Autodesk Inventor part; units mm, degrees
ref_plane "YZ Plane" through (0, 0, 0) normal (1, 0, 0) x (0, 1, 0)
ref_plane "XZ Plane" through (0, 0, 0) normal (0, 1, 0) x (-1, 0, 0)
ref_plane "XY Plane" through (0, 0, 0) normal (0, 0, 1) x (1, 0, 0)
sketch "Sketch1" plane through (0, 0, 0) normal (0, 1, 0) x (-1, 0, 0)
  line L0 (9.1683, 14.0813) -> (-48.6317, 14.0813)
  line L1 (-48.6317, 14.0813) -> (-48.6317, -63.9187)
  line L2 (-48.6317, -63.9187) -> (9.1683, -63.9187)
  line L3 (9.1683, -63.9187) -> (9.1683, 14.0813)
  point P0 (0, 0)
  dimension "d0" = 57.8
  dimension "d1" = 78
extrude "Extrusion1" add sketch "Sketch1" along normal blind 2
sketch "Sketch2" plane through (0, 2, 0) normal (0, 1, 0) x (1, 0, 0)
  line L0 (-9.1683, 63.9187) -> (-9.1683, -14.0813)
  line L1 (48.6317, 63.9187) -> (-9.1683, 63.9187)
  line L2 (-9.1683, -14.0813) -> (-1.1683, -14.0813)
  line L3 (-1.1683, -14.0813) -> (-1.1683, 63.9187)
  line L4 (-1.1683, 63.9187) -> (-9.1683, 63.9187)
  line L5 (-9.1683, 63.9187) -> (-9.1683, -14.0813)
  line L6 (48.6317, -14.0813) -> (48.6317, 63.9187)
  line L7 (48.6317, -14.0813) -> (40.6317, -14.0813)
  line L8 (40.6317, -14.0813) -> (40.6317, 63.9187)
  line L9 (40.6317, 63.9187) -> (48.6317, 63.9187)
  line L10 (48.6317, 63.9187) -> (48.6317, -14.0813)
  line L11 (1.2317, -14.0813) -> (1.2317, 63.9187)
  line L12 (-9.1683, -14.0813) -> (48.6317, -14.0813)
  line L13 (38.2317, -14.0813) -> (38.2317, 63.9187)
  line L14 (1.2317, -14.0813) -> (38.2317, -14.0813)
  line L15 (1.2317, 63.9187) -> (38.2317, 63.9187)
  point P0 (0, 0)
  dimension "d4" = 8
  dimension "d5" = 8
  dimension "d6" = 2.4
  dimension "d7" = 2.4
extrude "Extrusion2" add sketch "Sketch2" along normal blind 5.7 contours L1 L3 L2 L0 | L1 L13 L12 L11 | L1 L6 L7 L8
sketch "Sketch3" plane through (0, 7.7, 0) normal (0, 1, 0) x (1, 0, 0)
  circle A0 centre (9.7317, -0.0813) radius 1.35
  circle A1 centre (29.7317, -0.0813) radius 1.35
  line L0 (1.2317, 63.9187) -> (1.2317, -14.0813)
  circle A2 centre (9.7317, 49.9187) radius 1.35
  circle A3 centre (29.7317, 49.9187) radius 1.35
  line L1 (1.2317, -14.0813) -> (38.2317, -14.0813)
  point P0 (0, 0)
  dimension "d10" = 2.7
  dimension "d11" = 2.7
  dimension "d12" = 20
  dimension "d13" = 8.5
  dimension "d14" = 2.7
  dimension "d15" = 2.7
  dimension "d16" = 20
  dimension "d17" = 50
  dimension "d18" = 14
  dimension "d19" = 14
  dimension "d20" = 50
extrude "Extrusion3" cut sketch "Sketch3" against normal through all
sketch "Sketch4" plane through (0, 0, 0) normal (0, -1, 0) x (1, 0, 0)
  line L0 (8.7317, 14.0813) -> (8.7317, -13.9187)
  line L1 (8.7317, -13.9187) -> (-9.1683, -13.9187)
  line L2 (-9.1683, -35.9187) -> (8.7317, -35.9187)
  line L3 (8.7317, -35.9187) -> (8.7317, -63.9187)
  line L4 (8.7317, -63.9187) -> (30.7317, -63.9187)
  line L5 (30.7317, -63.9187) -> (30.7317, -35.9187)
  line L6 (30.7317, -35.9187) -> (48.6317, -35.9187)
  line L7 (48.6317, -13.9187) -> (30.7317, -13.9187)
  line L8 (30.7317, 14.0813) -> (30.7317, -13.9187)
  line L9 (30.7317, 14.0813) -> (8.7317, 14.0813)
  circle A0 centre (19.7317, 0.0813) radius 1.375
  circle A1 centre (19.7317, -49.9187) radius 1.375
  line L10 (48.6317, 14.0813) -> (48.6317, -63.9187)
  line L11 (-9.1683, 14.0813) -> (48.6317, 14.0813)
  line L12 (-9.1683, -13.9187) -> (-9.1683, -35.9187)
  line L13 (-9.1683, -63.9187) -> (-9.1683, 14.0813)
  line L14 (48.6317, -13.9187) -> (48.6317, -35.9187)
  line L15 (-9.1683, 14.0813) -> (48.6317, 14.0813)
  line L16 (48.6317, 14.0813) -> (48.6317, -63.9187)
  line L17 (48.6317, -63.9187) -> (-9.1683, -63.9187)
  line L18 (-9.1683, -63.9187) -> (-9.1683, 14.0813)
  point P0 (0, 0)
  point P1 (24.2887, -20.9845)
  point P2 (19.7317, -63.9187)
  dimension "d48" = 17.9
  dimension "d49" = 17.9
  dimension "d50" = 28
  dimension "d52" = 28
  dimension "d53" = 22
  dimension "d70" = 0
extrude "Extrusion4" add sketch "Sketch4" along normal blind 3 contours L0 L1 L13 L11 | L11 L10 L7 L8 | L2 L3 L17 L13 | L10 L17 L5 L6 | A0 | A1
sketch "Sketch5" plane through (24.7317, -3, 0.0813) normal (0, -1, 0) x (1, 0, 0)
  circle A0 centre (-5, 0) radius 1.375
  circle A1 centre (-5, 0) radius 1.375
  circle A2 centre (-5, -50) radius 1.375
  circle A3 centre (-5, -50) radius 1.375
  point P0 (-24.7317, -0.0813)
  dimension "d56" = 2.75
extrude "Extrusion5" cut sketch "Sketch5" against normal through all
sketch "Sketch6" plane through (0, 7.7, 0) normal (0, 1, 0) x (1, 0, 0)
  line L0 (12.2317, 63.9187) -> (27.2317, 63.9187)
  line L1 (27.2317, 63.9187) -> (27.2317, -14.0813)
  line L2 (27.2317, -14.0813) -> (12.2317, -14.0813)
  line L3 (12.2317, -14.0813) -> (12.2317, 63.9187)
  line L4 (38.2317, 63.9187) -> (1.2317, 63.9187)
  line L5 (1.2317, -14.0813) -> (38.2317, -14.0813)
  line L6 (48.6317, -14.0813) -> (48.6317, 63.9187)
  line L7 (-9.1683, 63.9187) -> (-9.1683, -14.0813)
  point P0 (0, 0)
  dimension "d59" = 0
  dimension "d60" = 0
  dimension "d61" = 21.4
  dimension "d62" = 21.4
extrude "Extrusion6" cut sketch "Sketch6" against normal blind 5.7
sketch "Sketch7" plane through (0, 7.7, 0) normal (0, 1, 0) x (1, 0, 0)
  line L0 (-9.1683, 63.9187) -> (-9.1683, -14.0813)
  line L1 (-1.1683, -14.0813) -> (1.2317, -14.0813)
  line L2 (-9.1683, 63.9187) -> (-1.1683, 63.9187)
  line L3 (-1.1683, 63.9187) -> (-1.1683, -14.0813)
  line L4 (-1.1683, -14.0813) -> (-9.1683, -14.0813)
  line L5 (-9.1683, -14.0813) -> (-9.1683, 63.9187)
  line L6 (48.6317, -14.0813) -> (48.6317, 63.9187)
  line L7 (40.6317, -14.0813) -> (40.6317, 63.9187)
  line L8 (48.6317, -14.0813) -> (40.6317, -14.0813)
  line L9 (40.6317, -14.0813) -> (40.6317, 63.9187)
  line L10 (40.6317, 63.9187) -> (48.6317, 63.9187)
  line L11 (48.6317, 63.9187) -> (48.6317, -14.0813)
  line L12 (1.2317, -14.0813) -> (1.2317, 63.9187)
  line L13 (1.2317, 63.9187) -> (4.4317, 63.9187)
  line L14 (4.4317, 63.9187) -> (4.4317, -14.0813)
  line L15 (4.4317, -14.0813) -> (1.2317, -14.0813)
  line L16 (1.2317, -14.0813) -> (1.2317, 63.9187)
  line L17 (38.2317, 63.9187) -> (38.2317, -14.0813)
  line L18 (38.2317, 63.9187) -> (35.0317, 63.9187)
  line L19 (35.0317, 63.9187) -> (35.0317, -14.0813)
  line L20 (35.0317, -14.0813) -> (38.2317, -14.0813)
  line L21 (38.2317, -14.0813) -> (38.2317, 63.9187)
  point P0 (0, 0)
  point P1 (38.2317, -14.0813)
  dimension "d71" = 3.2
  dimension "d72" = 3.2
extrude "Extrusion7" add sketch "Sketch7" along normal blind 29
fillet "Fillet6" radius 1.765 16 edges at (-1.1683, 19.35, 14.0813) (1.2317, 19.35, 14.0813) (1.2317, 36.7, -24.9187) (-1.1683, 36.7, -24.9187) (0.0317, 2, 14.0813) (38.2317, 36.7, -24.9187) (40.6317, 36.7, -24.9187) (38.2317, 19.35, 14.0813) (40.6317, 19.35, 14.0813) (39.4317, 2, 14.0813) (-1.1683, 19.35, -63.9187) (1.2317, 19.35, -63.9187) (38.2317, 19.35, -63.9187) (40.6317, 19.35, -63.9187) (39.4317, 2, -63.9187) (0.0317, 2, -63.9187)
properties part number "slider"
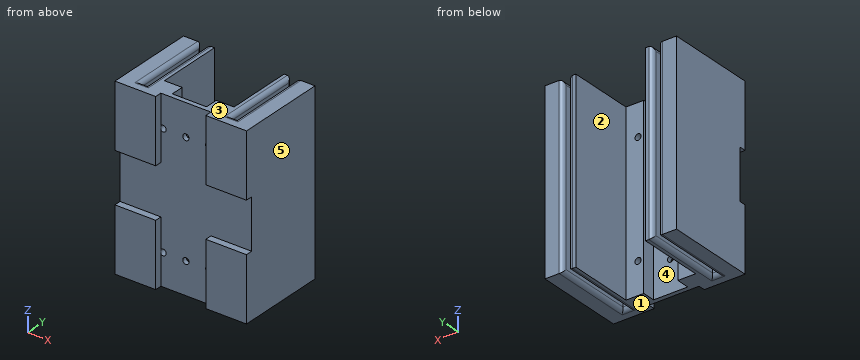
Geometry: final body of the model. Coordinates: model frame, mm. Face numbers are marked on the shaded views. A direction names the side the tool comes from. Round coordinates to 2 decimals unless told otherwise and drop trailing zeros. Order: outer loops, then holes, each group sorted by start corner. A loop starts at its lowest first (then second) coordinate and runs counter-clockwise, first axis right, second up. Notation, with made-up numbers: (9.5, -12) -> (22.5, -12) arc R28 ccw to (22.5, 26) -> close; hole circle Ø8 at (68, 6). An arc over 180 degrees is marked (long way). Put each result on its own line as item: value. Start each with the question number.
Q1. Section C-C on x = 25. Return the cut outline in (y, z).
Q2. Section A-A on y = 24. Return the cut outline in (x, z) (3 decimals).
Q3. Section B-B on z = -29.5. Return the cut outline in (x, y) (3 decimals), and give its area (3 significant figures).
Q4. Line query: probe 1 along X at (y, z) = (6.5, -44); probe 2 along X at (y, z) = (27, -49); probe 3 along Y at (x, z) = (5, -59). Output: solid intervals per line, ascending.
Q5. Reachability of the marked faces 1 and 2 from +Z, -Z, +X, -X, +Y, -Y: full face, straight path, thin tool, end or side. Return the list, or none.
Q6. Section D-D on z = -6.5. Return the cut outline in (x, y) (3 decimals).
Q7. Pull-direction query (X, two-part tool) for the marked faces 3, 4 and 5; classes: +X half, -X half, draft (parallel to the pull), parting line (faces both ways), or undercut.
Q8. First-contact query: pin 1 (2.5 mm diameter, centred on x = 9.73, z = -49.92, fed in from -Y); pin 2 (3 mm diameter, centred on x = 19.73, z = 0.08, fed in from -Y); pin 3 (12 mm diameter, centred on x = 21, z = -40, fed in from +Y); pin 4 (1.6 mm diameter, centred on x = 29.73, z = -49.92, fed in from -Y). Flat tips, straight axial feed; report the tip coordinate or a pass-through.
Ans:
1. outline: (0, -63.92) -> (2, -63.92) -> (2, 14.08) -> (0, 14.08) -> close
2. outline: (-9.168, -63.919) -> (-2.933, -63.919) arc R1.765 ccw to (-1.168, -62.154) -> (-1.168, 12.316) arc R1.765 ccw to (-2.933, 14.081) -> (-9.168, 14.081) -> close; (1.232, -62.154) arc R1.765 ccw to (2.997, -63.919) -> (4.432, -63.919) -> (4.432, 14.081) -> (2.997, 14.081) arc R1.765 ccw to (1.232, 12.316) -> close; (35.032, -63.919) -> (36.467, -63.919) arc R1.765 ccw to (38.232, -62.154) -> (38.232, 12.316) arc R1.765 ccw to (36.467, 14.081) -> (35.032, 14.081) -> close; (40.632, -62.154) arc R1.765 ccw to (42.397, -63.919) -> (48.632, -63.919) -> (48.632, 14.081) -> (42.397, 14.081) arc R1.765 ccw to (40.632, 12.316) -> close
3. outline: (-9.168, 0) -> (48.632, 0) -> (48.632, 36.7) -> (42.397, 36.7) arc R1.765 ccw to (40.632, 34.935) -> (40.632, 2) -> (38.232, 2) -> (38.232, 34.935) arc R1.765 ccw to (36.467, 36.7) -> (35.032, 36.7) -> (35.032, 7.7) -> (27.232, 7.7) -> (27.232, 2) -> (12.232, 2) -> (12.232, 7.7) -> (4.432, 7.7) -> (4.432, 36.7) -> (2.997, 36.7) arc R1.765 ccw to (1.232, 34.935) -> (1.232, 2) -> (-1.168, 2) -> (-1.168, 34.935) arc R1.765 ccw to (-2.933, 36.7) -> (-9.168, 36.7) -> close
3. area: 979 mm2
4. probe 1: x = -9.17 to -1.17, 1.23 to 12.23, 27.23 to 38.23, 40.63 to 48.63
4. probe 2: x = -9.17 to -1.17, 1.23 to 4.43, 35.03 to 38.23, 40.63 to 48.63
4. probe 3: y = -3 to 7.7
5. face 1: -Z, +X, -X, +Y, -Y
5. face 2: +Z, -Z, +Y
6. outline: (-9.168, -3) -> (8.732, -3) -> (8.732, 0) -> (30.732, 0) -> (30.732, -3) -> (48.632, -3) -> (48.632, 36.7) -> (42.397, 36.7) arc R1.765 ccw to (40.632, 34.935) -> (40.632, 2) -> (38.232, 2) -> (38.232, 34.935) arc R1.765 ccw to (36.467, 36.7) -> (35.032, 36.7) -> (35.032, 7.7) -> (27.232, 7.7) -> (27.232, 2) -> (12.232, 2) -> (12.232, 7.7) -> (4.432, 7.7) -> (4.432, 36.7) -> (2.997, 36.7) arc R1.765 ccw to (1.232, 34.935) -> (1.232, 2) -> (-1.168, 2) -> (-1.168, 34.935) arc R1.765 ccw to (-2.933, 36.7) -> (-9.168, 36.7) -> close
7. face 3: draft
7. face 4: undercut
7. face 5: +X half
8. pin 1: stops at y = -3
8. pin 2: stops at y = 0
8. pin 3: stops at y = 2
8. pin 4: passes through
